Check sheet for the modelled part. Datum: model origin and axes. Units: mm. Give positions to 0.01 mm unless a question says otherwise; leave off trailing zeros. Loops run counter-clockwise (first coordinate to the right, second up) from the corner with the lowest first, then second, coordinate; pieces in that order, holes last. Notation, with made-up numbers: M 89,73.25 L 133,73.25 A20 cw 133,87.25 Z; hole C 31.5,60.25 d8. An arc over 180 degrees is marked long. Use one line per item in the form item = value.
from build123d import *

# Parameters (mm, degrees)
SKETCH1_R           = 25.4
BOSS_EXTRUDE1_DEPTH = 152.4
SKETCH4_R           = 6.35
CUT_EXTRUDE1_DEPTH  = 175.26


with BuildPart() as part:
    # Sketch1 → Boss-Extrude1 (new body)
    with BuildSketch(Plane(origin=(0, 0, 0), x_dir=(1, 0, 0), z_dir=(0, 1, 0))):
        with Locations(Location((0, 0, 0), (0, 0, 90))):
            Circle(SKETCH1_R)
    extrude(amount=BOSS_EXTRUDE1_DEPTH)

    # Sketch2 → Revolve1 (revolve)
    with BuildSketch(Plane(origin=(0, 152.4, 0), x_dir=(1, 0, 0), z_dir=(0, 1, 0))):
        with BuildLine():
            Line((0, 25.4), (0, -25.4))
            ThreePointArc((0, -25.4), (-25.4, 0), (0, 25.4))
        make_face()
    revolve(axis=Axis((0, 152.4, -25.4), (0, 0, 1)))

    # Sketch4 → Cut-Extrude1 (cut)
    with BuildSketch(Plane.XZ):
        with Locations(Location((0, 0, 0), (0, 0, 270))):
            Circle(SKETCH4_R)
    extrude(amount=-CUT_EXTRUDE1_DEPTH, mode=Mode.SUBTRACT)


solid = part.part
1) Section check A-A (z = 0). Record the cut outline in (x, y).
Evaluation:
outline = M -25.4,0 L -6.35,0 L -6.35,175.26 L 6.35,175.26 L 6.35,0 L 25.4,0 L 25.4,152.4 A25.4 ccw -25.4,152.4 Z
2) Scan lines: line 1 (Z direction, x = -0.5, y = 37); line 2 (X direction, y = 102, z = 0); line 3 (Z direction, x = 5.5, y = 62). Record each from-to range of solid material in increasing order.
Evaluation:
line_1 = -25.4 to -6.33, 6.33 to 25.4
line_2 = -25.4 to -6.35, 6.35 to 25.4
line_3 = -24.8 to -3.17, 3.17 to 24.8
3) Section check B-B (x = 0). Record the cut outline in (y, z), then the cut area to 3 significant figures.
Evaluation:
outline = M 0,-25.4 L 152.4,-25.4 A25.4 ccw 152.4,25.4 L 0,25.4 L 0,6.35 L 175.26,6.35 L 175.26,-6.35 L 0,-6.35 Z
area = 6,530 mm^2
4) Section check D-D (x = 8). Record the cut outline in (y, z).
Evaluation:
outline = M 0,-24.11 L 152.4,-24.11 A24.11 ccw 152.4,24.11 L 0,24.11 Z
5) Release check for a two-part mould opening along Z. For faces 1 (the face through (5, 0, -5)), 2 (the face through (-3.86, 86.4, 5.04)), 3 (the face through (15.456, 75.133, 20.157)) record: pulls with the +Z half, pulls with the -Z half, needs draft (parallel to the pull), parting line crosses it, or undercut.
Evaluation:
face_1 = needs draft
face_2 = undercut
face_3 = parting line crosses it
6) Depth check by flat-ended pin: pin 1 Ø4 at (x, y) = (4.5, 143.5) entering from -Z; pin 2 Ø5 at (x, z) = (6, -6) entering from +Y; pin 3 Ø1 at (y, z) = (56.5, -9) entering from -X. Enter the tip coordinate at first touch or a pass-through.
Evaluation:
pin_1 = -25.28
pin_2 = 177.08
pin_3 = -23.94
7) Section check C-C (y = 150). Record the cut outline in (x, z), then the cut area to 3 significant figures.
Evaluation:
outline = C 0,0 d50.8; hole C 0,0 d12.7
area = 1,900 mm^2
